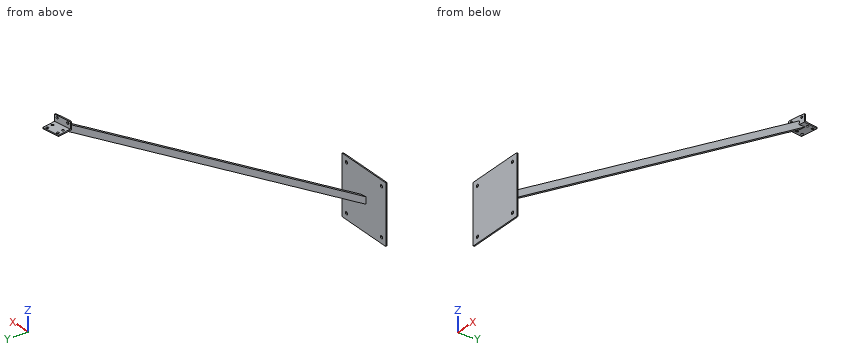
from build123d import *

# Parameters (mm, degrees)
BOSS_EXTRUDE1_DEPTH      = 60
BOSS_EXTRUDE2_DEPTH      = 2000
BOSS_EXTRUDE2_DEPTH_BACK = 20
SKETCH3_W                = 20
SKETCH3_H                = 20
SKETCH3_W_2              = 18
SKETCH3_H_2              = 18
CUT_EXTRUDE1_DEPTH       = 60
SKETCH7_W                = 200
SKETCH7_H                = 200
BOSS_EXTRUDE3_DEPTH      = 4
SKETCH8_W                = 109.20231627
SKETCH8_H                = 482.966945154
CUT_EXTRUDE3_DEPTH       = 1000
CUT_EXTRUDE4_REACH       = 1228.081
SKETCH9_R                = 3.999999996
CUT_EXTRUDE5_REACH       = 1228.081
SKETCH10_R               = 4.000000003
CUT_EXTRUDE6_REACH       = 1249.32
SKETCH11_R               = 5
FILLET1_R                = 2
FILLET2_R                = 2
BODY_MOVE_COPY1_ANGLE    = 9


with BuildPart() as part:
    # Sketch1 → Boss-Extrude1 (new body)
    with BuildSketch(Plane(origin=(0, 0, 0), x_dir=(0, 0, -1), z_dir=(1, 0, 0))):
        Polygon((0, 0), (0, 50), (-4, 50), (-4, 4), (-27, 4), (-27, 0), align=None)
    extrude(amount=BOSS_EXTRUDE1_DEPTH)

    # Sketch3 → Boss-Extrude2 (add, two sides: drawn at the far end of the back side and taken through both)
    with BuildSketch(Plane(origin=(0.734152256, 4.01424851, 2.317627458), x_dir=(0, -0.49999999999998884, 0.866025403784445), z_dir=(-0.1564344650402179, -0.8553631939770945, -0.4938441702975589)).offset(-BOSS_EXTRUDE2_DEPTH_BACK)):
        with Locations((0, -29.630650218)):
            Rectangle(SKETCH3_W, SKETCH3_H)
        with Locations((0, -29.630650218)):
            Rectangle(SKETCH3_W_2, SKETCH3_H_2, mode=Mode.SUBTRACT)
    extrude(amount=BOSS_EXTRUDE2_DEPTH + BOSS_EXTRUDE2_DEPTH_BACK)

    # Sketch5 → Cut-Extrude1 (cut)
    with BuildSketch(Plane.ZY):
        Polygon((4, 4), (4, 36.054903459), (38.781358344, 4), align=None)
    extrude(amount=-CUT_EXTRUDE1_DEPTH, mode=Mode.SUBTRACT)

    # Sketch7 → Boss-Extrude3 (add)
    with BuildSketch(Plane(origin=(-155.547262091, -982.086761679, 2e-09), x_dir=(0.9876883405962854, -0.15643446503298483, 2.850074130140158e-13), z_dir=(0.15643446503298483, 0.9876883405962854, -1.7994659856963007e-12))):
        with Locations((5.477031178, 566.441418592)):
            Rectangle(SKETCH7_W, SKETCH7_H)
    extrude(amount=BOSS_EXTRUDE3_DEPTH)

    # Sketch8 → Cut-Extrude3 (cut)
    with BuildSketch(Plane(origin=(-155.547262091, -982.086761679, 2e-09), x_dir=(0.9876883405962856, -0.15643446503298414, -2.6345368338963644e-10), z_dir=(-0.15643446503298414, -0.9876883405962856, 1.799719805411024e-12))):
        with Locations((4.33544583, -787.065663544)):
            Rectangle(SKETCH8_W, SKETCH8_H)
    extrude(amount=CUT_EXTRUDE3_DEPTH, mode=Mode.SUBTRACT)

    # Sketch9 → Cut-Extrude4 (cut, up to next)
    with BuildSketch(Plane(origin=(0, 0, 0), x_dir=(-1, 0, 0), z_dir=(0, 0, -1)), mode=Mode.PRIVATE) as cut_extrude4_sk1:
        with Locations((-50, 22)):
            Circle(SKETCH9_R)
    cut_extrude4_tool1 = extrude(cut_extrude4_sk1.sketch, amount=-CUT_EXTRUDE4_REACH, mode=Mode.PRIVATE) & part.part
    # Sketch9 → Cut-Extrude4 (cut, up to next)
    with BuildSketch(Plane(origin=(0, 0, 0), x_dir=(-1, 0, 0), z_dir=(0, 0, -1)), mode=Mode.PRIVATE) as cut_extrude4_sk2:
        with Locations((-10, 22)):
            Circle(SKETCH9_R)
    cut_extrude4_tool2 = extrude(cut_extrude4_sk2.sketch, amount=-CUT_EXTRUDE4_REACH, mode=Mode.PRIVATE) & part.part
    # Sketch9 → Cut-Extrude4 (cut, up to next)
    with BuildSketch(Plane(origin=(0, 0, 0), x_dir=(-1, 0, 0), z_dir=(0, 0, -1)), mode=Mode.PRIVATE) as cut_extrude4_sk3:
        with Locations((-10, 42)):
            Circle(SKETCH9_R)
    cut_extrude4_tool3 = extrude(cut_extrude4_sk3.sketch, amount=-CUT_EXTRUDE4_REACH, mode=Mode.PRIVATE) & part.part
    # Sketch9 → Cut-Extrude4 (cut, up to next)
    with BuildSketch(Plane(origin=(0, 0, 0), x_dir=(-1, 0, 0), z_dir=(0, 0, -1)), mode=Mode.PRIVATE) as cut_extrude4_sk4:
        with Locations((-50, 42)):
            Circle(SKETCH9_R)
    cut_extrude4_tool4 = extrude(cut_extrude4_sk4.sketch, amount=-CUT_EXTRUDE4_REACH, mode=Mode.PRIVATE) & part.part
    add(cut_extrude4_tool1.solids().sort_by_distance((50, 22, 0))[0], mode=Mode.SUBTRACT)
    add(cut_extrude4_tool2.solids().sort_by_distance((10, 22, 0))[0], mode=Mode.SUBTRACT)
    add(cut_extrude4_tool3.solids().sort_by_distance((10, 42, 0))[0], mode=Mode.SUBTRACT)
    add(cut_extrude4_tool4.solids().sort_by_distance((50, 42, 0))[0], mode=Mode.SUBTRACT)

    # Sketch10 → Cut-Extrude5 (cut, up to next)
    with BuildSketch(Plane.XZ, mode=Mode.PRIVATE) as cut_extrude5_sk1:
        with Locations(Location((50, 19, 0), (0, 0, 270))):
            Circle(SKETCH10_R)
    cut_extrude5_tool1 = extrude(cut_extrude5_sk1.sketch, amount=-CUT_EXTRUDE5_REACH, mode=Mode.PRIVATE) & part.part
    # Sketch10 → Cut-Extrude5 (cut, up to next)
    with BuildSketch(Plane.XZ, mode=Mode.PRIVATE) as cut_extrude5_sk2:
        with Locations(Location((10, 19, 0), (0, 0, 270))):
            Circle(SKETCH10_R)
    cut_extrude5_tool2 = extrude(cut_extrude5_sk2.sketch, amount=-CUT_EXTRUDE5_REACH, mode=Mode.PRIVATE) & part.part
    add(cut_extrude5_tool1.solids().sort_by_distance((50, 0, 19))[0], mode=Mode.SUBTRACT)
    add(cut_extrude5_tool2.solids().sort_by_distance((10, 0, 19))[0], mode=Mode.SUBTRACT)

    # Sketch11 → Cut-Extrude6 (cut, up to next)
    with BuildSketch(Plane(origin=(-155.547262091, -982.086761679, 2e-09), x_dir=(0.9876883405962856, -0.15643446503298414, -2.6345368338963665e-10), z_dir=(-0.15643446503298414, -0.9876883405962856, 1.7997198054110692e-12)), mode=Mode.PRIVATE) as cut_extrude6_sk1:
        with Locations((-74.522968646, -486.441418617)):
            Circle(SKETCH11_R)
    cut_extrude6_tool1 = extrude(cut_extrude6_sk1.sketch, amount=-CUT_EXTRUDE6_REACH, mode=Mode.PRIVATE) & part.part
    # Sketch11 → Cut-Extrude6 (cut, up to next)
    with BuildSketch(Plane(origin=(-155.547262091, -982.086761679, 2e-09), x_dir=(0.9876883405962856, -0.15643446503298414, -2.6345368338963665e-10), z_dir=(-0.15643446503298414, -0.9876883405962856, 1.7997198054110692e-12)), mode=Mode.PRIVATE) as cut_extrude6_sk2:
        with Locations((85.477031354, -486.441418617)):
            Circle(SKETCH11_R)
    cut_extrude6_tool2 = extrude(cut_extrude6_sk2.sketch, amount=-CUT_EXTRUDE6_REACH, mode=Mode.PRIVATE) & part.part
    # Sketch11 → Cut-Extrude6 (cut, up to next)
    with BuildSketch(Plane(origin=(-155.547262091, -982.086761679, 2e-09), x_dir=(0.9876883405962856, -0.15643446503298414, -2.6345368338963665e-10), z_dir=(-0.15643446503298414, -0.9876883405962856, 1.7997198054110692e-12)), mode=Mode.PRIVATE) as cut_extrude6_sk3:
        with Locations((85.477031354, -646.441418617)):
            Circle(SKETCH11_R)
    cut_extrude6_tool3 = extrude(cut_extrude6_sk3.sketch, amount=-CUT_EXTRUDE6_REACH, mode=Mode.PRIVATE) & part.part
    # Sketch11 → Cut-Extrude6 (cut, up to next)
    with BuildSketch(Plane(origin=(-155.547262091, -982.086761679, 2e-09), x_dir=(0.9876883405962856, -0.15643446503298414, -2.6345368338963665e-10), z_dir=(-0.15643446503298414, -0.9876883405962856, 1.7997198054110692e-12)), mode=Mode.PRIVATE) as cut_extrude6_sk4:
        with Locations((-74.522968646, -646.441418617)):
            Circle(SKETCH11_R)
    cut_extrude6_tool4 = extrude(cut_extrude6_sk4.sketch, amount=-CUT_EXTRUDE6_REACH, mode=Mode.PRIVATE) & part.part
    add(cut_extrude6_tool1.solids().sort_by_distance((-229.152729, -970.428801, -486.441419))[0], mode=Mode.SUBTRACT)
    add(cut_extrude6_tool2.solids().sort_by_distance((-71.122595, -995.458315, -486.441419))[0], mode=Mode.SUBTRACT)
    add(cut_extrude6_tool3.solids().sort_by_distance((-71.122595, -995.458315, -646.441419))[0], mode=Mode.SUBTRACT)
    add(cut_extrude6_tool4.solids().sort_by_distance((-229.152729, -970.428801, -646.441419))[0], mode=Mode.SUBTRACT)

    # Fillet1
    fillet1_edges = [part.edges().sort_by_distance(p)[0] for p in [
        (60, 50, 2),
        (60, 2, 27),
        (0, 2, 27),
        (0, 50, 2),
    ]]
    fillet(fillet1_edges, radius=FILLET1_R)

    # Fillet2
    fillet2_edges = [part.edges().sort_by_distance(p)[0] for p in [
        (-248.593627385, -965.324734939, -666.44141859),
        (-248.593627385, -965.324734938, -466.44141859),
        (-51.055959266, -996.611627945, -466.44141859),
        (-51.055959266, -996.611627945, -666.44141859),
    ]]
    fillet(fillet2_edges, radius=FILLET2_R)


with BuildPart() as part_1:
    # Body-Move/Copy1: read off the stored shape, not the designer's step
    # Body-Move/Copy1: moved
    add(part.part.moved(Location((1.9150449, 1006.4197144, 0))).rotate(Axis((0, 0, 0), (0, 0, 1)), BODY_MOVE_COPY1_ANGLE))


solid = part_1.part
Read the model definition and answer for the solid it produces. Units are mm, in the model's axes. Give positions to 0.01 mm unless a question says otherwise; leave off trailing zeros. Write each loop counter-clockwise with the first axis right and the second up, starting at its lowest first coordinate (ties: lowest second). Pieces come first, ordered by that corner, then holes. Notation, with made-up numbers: (-38.75, -33.75) - (0.25, -33.75) arc R30 ccw to (0.25, -10.75) - close; hole circle Ø1 at (7, 84.25). An arc over 180 degrees is marked (long way). Use CSV: the item, a comma, the result in double quotes. Start each with the question number.
Item 1: The part is cut by section C-C, the plane x = -192. Give the vertices of the cut face in (y, z), and give its area (3 significant figures).
Item 2: Consider line 1 (X direction, y = 729.5, z = -152.5); line 2 (Y direction, x = -82, z = -469); line 3 (Y direction, x = -138, z = -181). Determine where each line is inside the solid, lowest interval first.
Item 3: Flat-ended cylindrical pins translate along their axes: P1, Ø6, axis at x = -131, z = -301, coming from the -Y side; P2, Ø6.5, axis at x = -109.6, y = 1023.88, coming from the -Z side; P3, Ø16, axis at x = -230.07, z = -486.44, coming from the +Y side; P4, Ø9, axis at x = -112.73, y = 1043.63, coming from the +Z side. Find the tip coordinate at first contact, or state that the pin passes through.
Item 4: The part is cut by section B-B, the plane z = -456. Give the vertices of the cut face in (x, y), and give its area (3 significant figures).
Item 5: The part is cut by section A-A, the plane y = 899. Give the vertices of the cut face in (x, z), and give its area (3 significant figures).
Taken from the geometry:
1,outline,"(0, -666.44) - (4, -666.44) - (4, -466.44) - (0, -466.44) - close"
1,area,"800 mm2"
2,line 1,"-142.32 to -141.32, -123.26 to -122.25"
2,line 2,"0 to 4"
2,line 3,"659.45 to 661.47, 697.92 to 699.95"
3,P1,"y = 444.84"
3,P2,"through"
3,P3,"y = 4"
3,P4,"z = 4"
4,outline,"(-155.45, 214.93) - (-154.61, 174.57) - (-134.61, 177.73) - (-135.45, 218.1) - close; hole (-154.41, 213.07) - (-153.65, 176.74) - (-135.65, 179.59) - (-136.41, 215.92) - close"
4,area,"154 mm2"
5,outline,"(-139.16, -67.39) - (-119.24, -69.19) - (-117.44, -46.26) - (-137.36, -44.46) - close; hole (-138.07, -66.33) - (-120.14, -67.95) - (-118.52, -47.31) - (-136.45, -45.69) - close"
5,area,"87.4 mm2"
